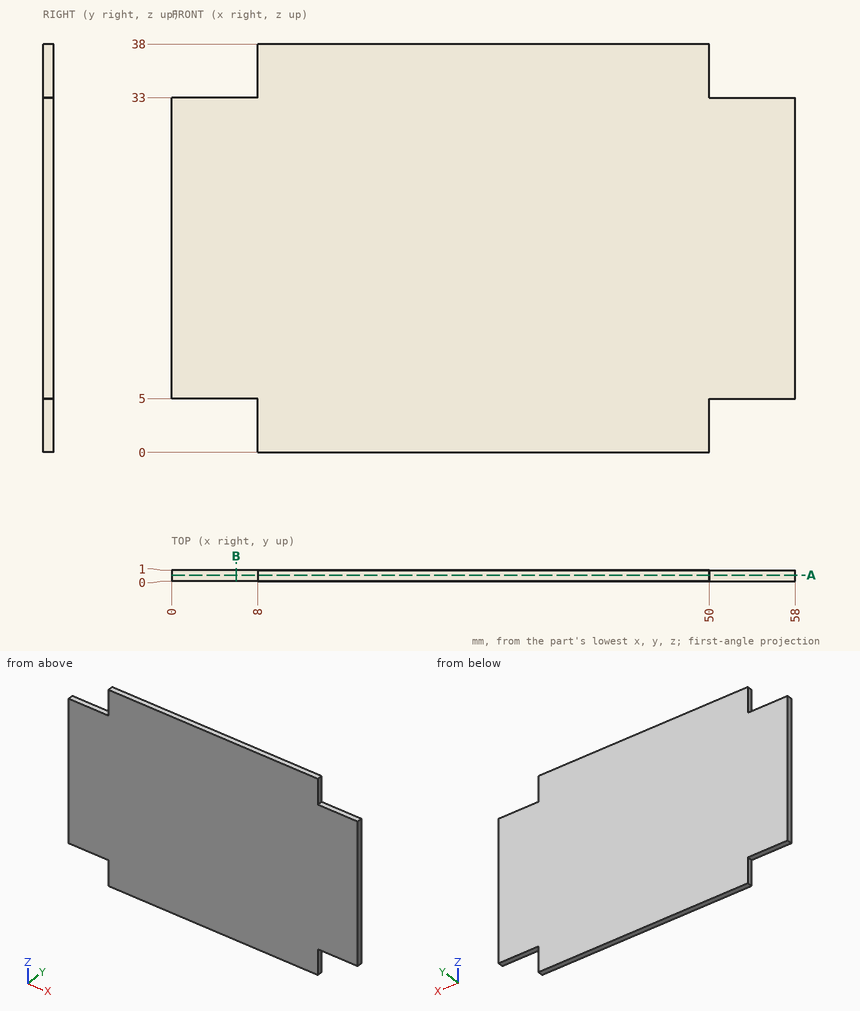
Verification items for this drawing (mm, ordinates from the low corner). Give positions to 0.01 mm unless a question says otherwise; leave off trailing zeros. Write each loop counter-clockwise with the first axis right and the second up, starting at its lowest first coordinate (ties: lowest second). Pieces come first, ordered by that corner, then holes.
1) Go/stop test with flat-tipped pins: pin 1 Ø0.5 at (y, z) = (0.5, 35.5) entering from -X; pin 2 Ø0.5 at (x, y) = (5.5, 0.5) entering from +Z; pin 3 Ø0.5 at (x, y) = (52, 0.5) entering from -Z. Record where each tip stops, or that it passes through.
Values follow:
pin 1: stops at x = 8
pin 2: stops at z = 33
pin 3: stops at z = 5
2) Cross-section at A-A (y = 0.55). Record the boundary of the cut face in (x, z), plus the area to 3 significant figures.
Values follow:
outline: (0, 5) - (8, 5) - (8, 0) - (50, 0) - (50, 5) - (58, 5) - (58, 33) - (50, 33) - (50, 38) - (8, 38) - (8, 33) - (0, 33) - close
area: 2,040 mm2
3) Thickness scan on line 1 (Z direction, x = 51.5, y = 0.3); line 2 (X direction, y = 0.85, z = 36). Record the ranges inside material, lowest first.
Values follow:
line 1: z = 5 to 33
line 2: x = 8 to 50
4) Cross-section at B-B (x = 6). Record the boundary of the cut face in (y, z), plus the area to 3 significant figures.
Values follow:
outline: (0, 5) - (1, 5) - (1, 33) - (0, 33) - close
area: 28.0 mm2
